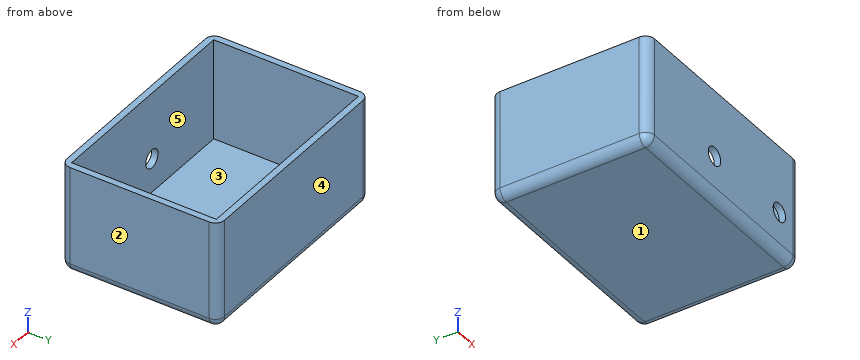
Autodesk Inventor part; units mm, degrees
ref_plane "YZ Plane" through (0, 0, 0) normal (1, 0, 0) x (0, 1, 0)
ref_plane "XZ Plane" through (0, 0, 0) normal (0, 1, 0) x (-1, 0, 0)
ref_plane "XY Plane" through (0, 0, 0) normal (0, 0, 1) x (1, 0, 0)
sketch "Sketch1" plane through (0, 0, 0) normal (0, 0, 1) x (1, 0, 0)
  line L0 (0, 0) -> (46, 0)
  line L1 (46, 0) -> (46, 31.5)
  line L2 (46, 31.5) -> (0, 31.5)
  line L3 (0, 31.5) -> (0, 0)
  line L4 (-1.4, 32.9) -> (47.4, 32.9)
  line L5 (47.4, 32.9) -> (47.4, -1.4)
  line L6 (47.4, -1.4) -> (-1.4, -1.4)
  line L7 (-1.4, -1.4) -> (-1.4, 32.9)
  dimension "d0" = 46
  dimension "d1" = 31.5
  dimension "d2" = 1.4
extrude "Extrusion1" add sketch "Sketch1" along normal blind 22
sketch "Sketch2" plane through (0, 0, 0) normal (0, 0, -1) x (-1, 0, 0)
  line L0 (1.4, -1.4) -> (1.4, 32.9)
  line L1 (-47.4, -1.4) -> (1.4, -1.4)
  line L2 (1.4, 32.9) -> (-47.4, 32.9)
  line L3 (-47.4, 32.9) -> (-47.4, -1.4)
  point P0 (0, 0)
extrude "Extrusion2" add sketch "Sketch2" along normal blind 1.4
sketch "Sketch3" plane through (-1.4, -1.4, 22) normal (0, -1, 0) x (1, 0, 0)
  circle A0 centre (21.4, -14.5673) radius 2
  line L0 (1.4, -22) -> (1.4, 0)
  circle A1 centre (42.4, -14.5673) radius 2
  line L1 (47.4, -22) -> (47.4, 0)
  dimension "d7" = 4
  dimension "d8" = 20
  dimension "d9" = 4
  dimension "d10" = 5
extrude "Extrusion3" cut sketch "Sketch3" against normal blind 1.4
fillet "Fillet1" radius 2 8 edges at (-1.4, -1.4, 10.3) (47.4, -1.4, 10.3) (47.4, 32.9, 10.3) (-1.4, 32.9, 10.3) (47.4, 15.75, -1.4) (23, -1.4, -1.4) (-1.4, 15.75, -1.4) (23, 32.9, -1.4)
properties part number "relay-housing"
Design review of the part built by this model. Coordinates are the model's own, in mm. Face numbers are marked on the shaded views. A direction names the side the tool comes from. Coordinates: 2 decimals unless noted, no trailing zeros. Loops run counter-clockwise (first coordinate to the right, second up) from the corner with the lowest first, then second, coordinate; pieces in that order, holes last. Notation, with made-up numbers: M 32.25,-23 L 72.25,-23 A13 cw 72.25,-3 Z; hole C 28,86.25 d2. An arc over 180 degrees is marked long. One line per question, with ' | ' between items.
(1) We need section B-B (x = 20). Give the boundary of the cut face in (y, z), and give its area (3 significant figures).
Filled in:
outline: M -1.4,0.6 A2 ccw 0.6,-1.4 L 30.9,-1.4 A2 ccw 32.9,0.6 L 32.9,22 L 31.5,22 L 31.5,0 L 0,0 L 0,5.43 L -1.4,5.43 Z; M -1.4,9.43 L 0,9.43 L 0,22 L -1.4,22 Z | area: 102 mm^2
(2) For pin 1 Ø1.5 at (x, y) = (29.5, 29.5) entering from +Z, flat-tipped, find the tip position at first contact; note if it passes through.
Filled in:
pin 1: stops at z = 0
(3) We need section D-D (x = 7.5). Give the boundary of the cut face in (y, z), and give its area (3 significant figures).
Filled in:
outline: M -1.4,0.6 A2 ccw 0.6,-1.4 L 30.9,-1.4 A2 ccw 32.9,0.6 L 32.9,22 L 31.5,22 L 31.5,0 L 0,0 L 0,22 L -1.4,22 Z | area: 108 mm^2
(4) Draft analysis for pull direction X (two halves, no side actions). For the marked faces 1, 2 and 3, state which applies: released by +X, released by -X, zero draft, split by the parting line, or undercut.
Filled in:
face 1: zero draft | face 2: released by +X | face 3: undercut
(5) Machinability: for the marked faces 4 and 5, which of the approach directions +Z, -Z, +X, -X, +Y, -Y give a long, thin tool a straight path to every point of the face, cutting with its end or side? Answer none if there is none.
Filled in:
face 4: +Z, -Z, +X, -X, +Y | face 5: +Z
(6) We need section C-C (y = 13.5). Give the boundary of the cut face in (x, z).
Filled in:
outline: M -1.4,0.6 A2 ccw 0.6,-1.4 L 45.4,-1.4 A2 ccw 47.4,0.6 L 47.4,22 L 46,22 L 46,0 L 0,0 L 0,22 L -1.4,22 Z
(7) We need section A-A (z = 3.5). Give the boundary of the cut face in (x, y), and give its area (3 significant figures).
Filled in:
outline: M -1.4,0.6 A2 ccw 0.6,-1.4 L 45.4,-1.4 A2 ccw 47.4,0.6 L 47.4,30.9 A2 ccw 45.4,32.9 L 0.6,32.9 A2 ccw -1.4,30.9 Z; hole M 0,0 L 46,0 L 46,31.5 L 0,31.5 Z | area: 221 mm^2
(8) Wall thickness on probe 1 along X at (y, z) = (13.5, 7.5); probe 2 along Y at (x, z) = (16.5, 2); probe 3 along Z at (x, y) = (8, 9): over which ranges is each line inside the solid? List them lowest first.
Filled in:
probe 1: x = -1.4 to 0, 46 to 47.4 | probe 2: y = -1.4 to 0, 31.5 to 32.9 | probe 3: z = -1.4 to 0
